Can you work these out from the model? Positions are in its coordinate system, mm. A direction names the side the tool comes from. Coordinates: 2 decimals unless noted, no trailing zeros. Order: outer loops, then holes, each group sorted by start corner. A loop starts at its lowest first (then second) coordinate and runs counter-clockwise, first axis right, second up. Notation, with made-up numbers: (12, 79.5) -> (63, 79.5) arc R29 ccw to (63, 114.5) -> close; hole circle Ø6 at (-24, 81). An arc over 180 degrees is marked (long way). Answer in a Markdown table with one row per item.
```python
from build123d import *

# Parameters (mm, degrees)
BOSS_EXTRUDE1_DEPTH = 50.8
SKETCH3_W           = 103.793513641
SKETCH3_H           = 1.78121028
CUT_EXTRUDE1_DEPTH  = 2.54


with BuildPart() as part:
    # Sketch1 → Boss-Extrude1 (new body)
    with BuildSketch(Plane(origin=(0, -33.456799282, 0), x_dir=(1, 0, 0), z_dir=(0, 1, 0))):
        with BuildLine():
            Line((-527.50657757, -80.842567675), (-695.232596141, -28.656691245))
            ThreePointArc((-695.232596141, -28.656691245), (-714.028086723, 7.11747239), (-678.253923088, 25.912962972))
            ThreePointArc((-678.253923088, 25.912962972), (-674.077147403, 17.963148831), (-682.026961544, 13.786373146))
            ThreePointArc((-682.026961544, 13.786373146), (-697.926589826, 5.432821776), (-689.573038456, -10.466806506))
            Line((-689.573038456, -10.466806506), (-533.973609712, -58.87964448))
            Line((-533.973609712, -58.87964448), (-528.314052027, -40.689759741))
            Line((-528.314052027, -40.689759741), (-516.187462201, -44.462798197))
            Line((-516.187462201, -44.462798197), (-527.50657757, -80.842567675))
        make_face()
    extrude(amount=BOSS_EXTRUDE1_DEPTH)

    # Sketch3 → Cut-Extrude1 (cut)
    with BuildSketch(Plane(origin=(-69.492010407, 0, 223.348136035), x_dir=(0.9548495925978474, 0, 0.2970896422222171), z_dir=(-0.29708964222221707, 0, 0.9548495925978473))):
        with Locations((-603.432198215, 0.071200718)):
            Rectangle(SKETCH3_W, SKETCH3_H)
    extrude(amount=-CUT_EXTRUDE1_DEPTH, mode=Mode.SUBTRACT)


solid = part.part
```
(1) Suppose I cut it at A-A (x = -685.8). Please give me the cut outline in (y, z).
Response values:
| item | result |
|---|---|
| outline | (-33.46, -27.19) -> (17.34, -27.19) -> (17.34, -14.36) -> (-33.46, -14.36) -> close; (-33.46, 11.64) -> (17.34, 11.64) -> (17.34, 31.59) -> (0.96, 31.59) -> (0.96, 28.93) -> (-0.82, 28.93) -> (-0.82, 31.59) -> (-33.46, 31.59) -> close |
(2) I need wall thicknesses on line 1 (Z direction, x = -694, y = -27); line 2 (Z direction, x = -674.5, y = -17.5); line 3 (X direction, y = -6, z = -7.5). Which ranges of each line are inside material? Lowest first, please. Write a range as [from, to].
Response values:
| item | result |
|---|---|
| line 1 | [-26.27, -11.36], [8.04, 29.04] |
| line 2 | [-22.77, -16.93], [15.16, 35.11] |
| line 3 | [-713.91, -697.08] |
(3) Suppose I cut it at B-B (x = -651.5). Please give me the cut outline in (y, z), and give its area (3 significant figures).
Response values:
| item | result |
|---|---|
| outline | (-33.46, 22.31) -> (17.34, 22.31) -> (17.34, 42.26) -> (0.96, 42.26) -> (0.96, 39.6) -> (-0.82, 39.6) -> (-0.82, 42.26) -> (-33.46, 42.26) -> close |
| area | 1,010 mm2 |
(4) Will these pins go through, and if not, where does the flat tip stop? pin 1 Ø1 at (x, y) = (-655.5, -12) entering from +Z; pin 2 Ø10 at (x, y) = (-630, -26.5) entering from +Z; pin 3 Ø12 at (x, y) = (-538, 8) entering from +Z.
Response values:
| item | result |
|---|---|
| pin 1 | z = 41.17 |
| pin 2 | z = 50.51 |
| pin 3 | z = 79.44 |
(5) Suppose I cut it at D-D (z = 67.5). Please give me the cut outline in (x, y), and give its area (3 significant figures).
Response values:
| item | result |
|---|---|
| outline | (-570.39, -33.46) -> (-523.36, -33.46) -> (-523.36, 17.34) -> (-570.39, 17.34) -> close |
| area | 2,390 mm2 |
(6) On a 3-axis mill with a long thin cutter (end or side, diameter ignored), from which of +Z, -Z, +X, -X, +Y, -Y can I reach the whole of each face in a straight line? I mean faces 1 (the flat face through (-531.183, -8.412, 49.912)), 2 (the flat face through (-630, -33.457, 35)). Say none if no direction works.
Response values:
| item | result |
|---|---|
| face 1 | -Z, +Y, -Y |
| face 2 | +Z, -Z, +X, -X, -Y |
(7) Suppose I cut it at C-C (y = 12.5). Please give me the cut outline in (x, z) (3 decimals), and give its area (3 significant figures).
Response values:
| item | result |
|---|---|
| outline | (-695.233, 28.657) arc R28.575 ccw to (-678.254, -25.913) arc R6.35 ccw to (-682.027, -13.786) arc R12.7 cw to (-689.573, 10.467) -> (-533.974, 58.88) -> (-528.314, 40.69) -> (-516.187, 44.463) -> (-527.507, 80.843) -> close |
| area | 4,680 mm2 |
(8) We'd pull the mould along Z, two halves only. Please class faces 3 (the cylindrical face through (-674.037, -8.412, -18.097)), 4 (the flat face through (-521.77, -8.41, 62.4)), 5 (the flat face through (-522.34, -8.41, 42.55)): +Z half, -Z half, draft (parallel to the pull), parting line (faces both ways), or undercut.
Response values:
| item | result |
|---|---|
| face 3 | undercut |
| face 4 | +Z half |
| face 5 | -Z half |
